```python
from build123d import *

# Parameters (mm, degrees)
BOSS_EXTRUDE1_DEPTH                            = 6.35
F_1_4_CLEARANCE_HOLE2_D                        = 7.14248
CBORE_FOR_6_SOCKET_HEAD_CAP_SCREW1_D           = 4.3053
CBORE_FOR_6_SOCKET_HEAD_CAP_SCREW1_CBORE_D     = 7.14502
CBORE_FOR_6_SOCKET_HEAD_CAP_SCREW1_CBORE_DEPTH = 3.5052


with BuildPart() as part:
    # Sketch1 → Boss-Extrude1 (new body)
    with BuildSketch(Plane(origin=(0, 0, 0), x_dir=(1, 0, 0), z_dir=(0, 1, 0))):
        Polygon((0, 12.7), (88.9, 12.7), (107.95, 6.35), (107.95, -6.35), (-19.05, -6.35), (-19.05, 6.35), align=None)
    extrude(amount=BOSS_EXTRUDE1_DEPTH)

    # 1/4 Clearance Hole2 (through all)
    with Locations(Plane(origin=(0, 0, 0), x_dir=(-1, 0, 0), z_dir=(0, -1, 0))):
        with Locations((-101.6, 0), (12.7, 0)):
            Hole(F_1_4_CLEARANCE_HOLE2_D / 2)

    # CBORE for #6 Socket Head Cap Screw1 (through all)
    with Locations(Plane(origin=(0, 0, 0), x_dir=(-1, 0, 0), z_dir=(0, -1, 0))):
        with Locations((-80.9625, 6.35), (-7.9375, 6.35)):
            CounterBoreHole(CBORE_FOR_6_SOCKET_HEAD_CAP_SCREW1_D / 2, CBORE_FOR_6_SOCKET_HEAD_CAP_SCREW1_CBORE_D / 2, CBORE_FOR_6_SOCKET_HEAD_CAP_SCREW1_CBORE_DEPTH)


solid = part.part
```
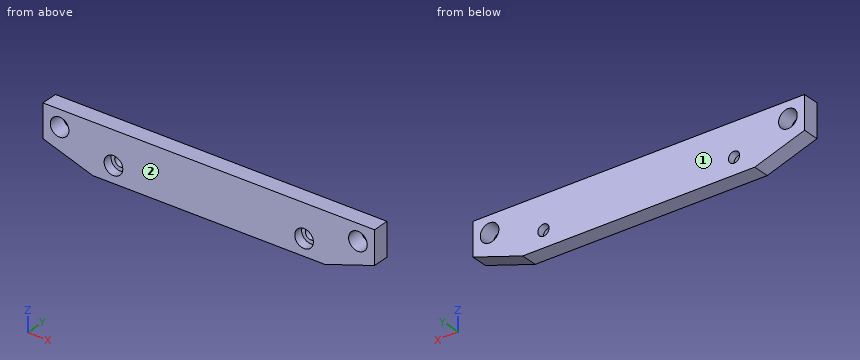
CAD build for the part. Positions are in the model's coordinates, mm. Face numbers are marked on the shaded views. Coordinates: 2 decimals unless noted, no trailing zeros. Order: outer loops, then holes, each group sorted by start corner. A loop starts at its lowest first (then second) coordinate and runs counter-clockwise, first axis right, second up.
(1) Saw through at C-C, the plane x = 101.6. Write the cut outline in (y, z).
Solution:
outline: (0, -8.47) - (6.35, -8.47) - (6.35, -3.57) - (0, -3.57) - close; (0, 3.57) - (6.35, 3.57) - (6.35, 6.35) - (0, 6.35) - close
(2) Pin check, flat tips, straight feed: pin 1 Ø5.5 at (x, z) = (7.94, -6.35) entering from -Y; pin 2 Ø8 at (x, z) = (48.5, 2.5) entering from -Y; pin 3 Ø5.5 at (x, z) = (101.6, 0) entering from -Y. Stop position of each tip, or through.
Solution:
pin 1: stops at y = 3.51
pin 2: stops at y = 0
pin 3: passes through
(3) Saw through at A-A, the plane z = 0. Write the cut outline in (x, y), and give its area (3 significant figures).
Solution:
outline: (-19.05, 0) - (-16.27, 0) - (-16.27, 6.35) - (-19.05, 6.35) - close; (-9.13, 0) - (98.03, 0) - (98.03, 6.35) - (-9.13, 6.35) - close; (105.17, 0) - (107.95, 0) - (107.95, 6.35) - (105.17, 6.35) - close
area: 716 mm2
(4) Mould opens along Y. For the marked faces 1 and 2 say: released by +Y, released by -Y, zero draft, split by the parting line, or undercut.
Solution:
face 1: released by +Y
face 2: released by -Y
(5) Drill centre lines: L1, parallel to X at y = 3.75, z = -6; L2, parallel to X at y = 1.25, z = -2.5; L3, parallel to Z at x = 6.5, y = 4.25. Where is each one in solid material? Low to high.
Solution:
L1: x = -19.05 to 5.81, 10.06 to 78.84, 83.09 to 107.95
L2: x = -19.05 to -15.25, -10.15 to 99.05, 104.15 to 107.95
L3: z = -12.7 to -7.95, -4.75 to 6.35
(6) Saw through at B-B, the plane y = 2. Count the separate pieces of the cut face and the enclosed holes in it, and give its area (3 significant figures).
Solution:
separate pieces: 1
enclosed holes: 4
area: 2,140 mm2
